```python
from build123d import *

# Parameters (mm, degrees)
SKETCH_1_R      = 2.5
EXTRUDE_1_DEPTH = 5
SKETCH_2_R      = 3
EXTRUDE_2_DEPTH = 34
EXTRUDE_START   = 24
SKETCH_3_R      = 2.5
EXTRUDE_3_DEPTH = 24
SKETCH_4_R      = 2
EXTRUDE_4_DEPTH = 12


with BuildPart() as part:
    # 草图1 → 凸台-拉伸1 (new body)
    with BuildSketch(Plane.XY):
        Circle(SKETCH_1_R)
    extrude(amount=EXTRUDE_1_DEPTH)

    # 草图2 → 凸台-拉伸2 (add)
    with BuildSketch(Plane(origin=(0, 0, 0), x_dir=(-1, 0, 0), z_dir=(0, 0, -1))):
        Circle(SKETCH_2_R)
    extrude(amount=EXTRUDE_2_DEPTH)

    # 草图3 → 凸台-拉伸3 (add)
    with BuildSketch(Plane(origin=(0, 0, -34), x_dir=(-1, 0, 0), z_dir=(0, 0, -1)).offset(EXTRUDE_START)):
        with Locations(Location((0, 0, 0), (0, 0, 180))):
            Circle(SKETCH_3_R)
    extrude(amount=-EXTRUDE_3_DEPTH)

    # 草图4 → 凸台-拉伸4 (add)
    with BuildSketch(Plane(origin=(0, 0, -58), x_dir=(-1, 0, 0), z_dir=(0, 0, -1))):
        Circle(SKETCH_4_R)
    extrude(amount=EXTRUDE_4_DEPTH)


solid = part.part
```
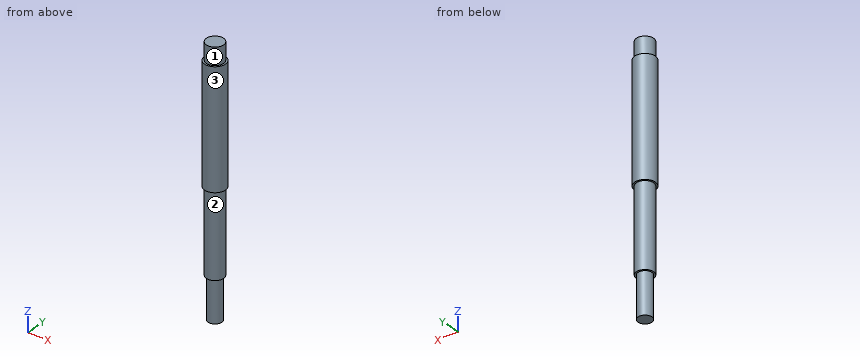
Read the model definition and answer for the solid it produces. Units are mm, in the model's axes. Face numbers are marked on the shaded views. A direction names the side the tool comes from. Give positions to 0.01 mm unless a question says otherwise; leave off trailing zeros. Write each loop counter-clockwise with the first axis right and the second up, starting at its lowest first coordinate (ties: lowest second). Pieces come first, ordered by that corner, then holes. Notation, with made-up numbers: M 60,28.25 L 114,28.25 A24 cw 114,40.25 Z; hole C 83,59.5 d3. An arc over 180 degrees is marked long. Put each result on its own line as item: value. Start each with the question number.
1. Which of the six approach directions +Z, -Z, +X, -X, +Y, -Y give full straight-line access (tool end or side, diameter ignored) to the marked faces 1, 2 and 3?
2. The part is cut by section D-D, the plane z = -51.5. Give the vertices of the cut face in (x, y).
3. Consider line 1 along Z through (x, y) = (-1.75, -2.3); line 2 along Y through (x, z) = (0.1, -6); line 3 along Z through (x, y) = (-0.6, 2.1). Determine where each line is inside the solid, lowest interval first.
4. Each of these flat-tipped pins is pushed along its axis until it touches: pin 1 Ø2 at (x, z) = (-2, -15) entering from +Y; pin 2 Ø1 at (x, z) = (-0.5, -46.5) entering from +Y; pin 3 Ø2 at (x, z) = (-0.5, -3) entering from +Y. Where does it stop, or does it pass through?
5. The part is cut by section A-A, the plane y = 0. Give the vertices of the cut face in (x, z).
6. The part is cut by section C-C, the plane z = -33. Give the vertices of the cut face in (x, y).
Final values:
1. face 1: +Z
1. face 2: -Z
1. face 3: +Z, -Z
2. outline: C 0,0 d5
3. line 1: z = -34 to 0
3. line 2: y = -3 to 3
3. line 3: z = -58 to 5
4. pin 1: stops at y = 2.83
4. pin 2: stops at y = 2.5
4. pin 3: stops at y = 3
5. outline: M -3,-34 L -2.5,-34 L -2.5,-58 L -2,-58 L -2,-70 L 2,-70 L 2,-58 L 2.5,-58 L 2.5,-34 L 3,-34 L 3,0 L 2.5,0 L 2.5,5 L -2.5,5 L -2.5,0 L -3,0 Z
6. outline: C 0,0 d6
